Read the model definition and answer for the solid it produces. Units are mm, in the model's axes. A direction names the side the tool comes from. Coordinates: 2 decimals unless noted, no trailing zeros. Loops run counter-clockwise (first coordinate to the right, second up) from the corner with the lowest first, then second, coordinate; pieces in that order, holes last. Notation, with made-up numbers: (-38.5, 63) -> (-34.5, 63) arc R25 ccw to (-34.5, 81) -> close; hole circle Ø6 at (-4, 57). An arc over 180 degrees is marked (long way). Answer as a JSON object with one key per item and string values. Group by question number.
Q1. Straight lines are drawn through the part: line 1 along Z through (x, y) = (2.5, 3.5); line 2 along Z through (x, y) = (0, 0.5); line 3 along Z through (x, y) = (0, 4.85). For each, find the intervals that lie inside material, in ascending order. Write a range as [from, to].
Q2. The part is cut by section A-A on x = 0. Write down the section's boundary in (y, z).
Q3. The part is cut by section B-B on z = -6.5. Write down the section's boundary in (x, y).
Q4. Determine the mould class of faces 1 (the cylindrical face through (-0.404, 4.021, -9.574)), 2 (the flat face through (3, 5.5, 5)), 3 (the flat face through (4, 2, 1)) for opening direction X: released by +X, released by -X, zero draft, split by the parting line, or undercut.
Q5. Each of these flat-tipped pins is pushed along its axis until it touches: P1, Ø3, axis at x = -1.5, z = 8.5, coming from the -Y side; P2, Ø1, axis at x = 0.5, z = 0, coming from the -Y side; P3, Ø2.5, axis at x = 1.5, z = -6, coming from the -Y side; P4, Ø1.8, axis at x = 0, z = -6.5, coming from the -Y side (1 decimal). Where does it stop, or does it pass through?
Q6. For faces 4 (the flat face through (0, 0, -4)), 5 (the flat face through (0, -4, 7)), 6 (the flat face through (0, 4.5, 9.5)), determine the directions among +Z, -Z, +X, -X, +Y, -Y from which every point of the face is accessible in a straight line to the end or side of a thin tool.
Autodesk Inventor part; units mm, degrees
ref_plane "YZ Plane" through (0, 0, 0) normal (1, 0, 0) x (0, 1, 0)
ref_plane "XZ Plane" through (0, 0, 0) normal (0, 1, 0) x (-1, 0, 0)
ref_plane "XY Plane" through (0, 0, 0) normal (0, 0, 1) x (1, 0, 0)
sketch "Sketch1" plane through (0, 0, 0) normal (0, 1, 0) x (-1, 0, 0)
  line L0 (0, 10) -> (0, 10)
  line L1 (-4, 6) -> (-4, -6)
  line L2 (0, -10) -> (0, -10)
  line L3 (4, -6) -> (4, 6)
  line L4 (4, 10) -> (-4, -10) construction
  line L5 (-4, 10) -> (4, -10) construction
  circle A0 centre (0, -6.5) radius 1.5
  arc A1 (0, -10) -> (4, -6) centre (0, -6) ccw
  arc A2 (-4, -6) -> (0, -10) centre (0, -6) ccw
  arc A3 (4, 6) -> (0, 10) centre (0, 6) ccw
  arc A4 (0, 10) -> (-4, 6) centre (0, 6) ccw
  point P0 (0, 0)
  dimension "d0" = 8
  dimension "d1" = 20
  dimension "d2" = 3
  dimension "d3" = 3.5
  dimension "d4" = 4
extrude "Extrusion1" add sketch "Sketch1" along normal blind 5.5
sketch "Sketch2" plane through (0, 0, 0) normal (0, -1, 0) x (1, 0, 0)
  circle A0 centre (0, -6.5) radius 1.5 construction
  line L0 (-4, -6) -> (-4, 6) construction
  arc A1 (-4, -6) -> (4, -6) centre (0, -6) ccw construction
  line L1 (4, 6) -> (4, -6) construction
  arc A2 (4, 6) -> (-4, 6) centre (0, 6) ccw construction
  arc A3 (4, 6) -> (-4, 6) centre (0, 6) ccw
  arc A4 (4, 6) -> (-4, 6) centre (0, 5.2831) ccw
  point P0 (0, 0)
extrude "Extrusion2" cut sketch "Sketch2" against normal blind 4.5
sketch "Sketch4" plane through (0, 0, 0) normal (0, -1, 0) x (1, 0, 0)
  arc A0 (4, 6) -> (-4, 6) centre (0, 5.2831) ccw
  line L0 (-4, -6) -> (-4, 6)
  arc A1 (-4, -6) -> (4, -6) centre (0, -6) ccw
  line L1 (4, 6) -> (4, -6)
  circle A2 centre (0, -6.5) radius 1.5
  point P0 (0, 0)
extrude "Extrusion3" add sketch "Sketch4" along normal blind 4
sketch "Sketch6" plane through (0, -4, 0) normal (0, -1, 0) x (1, 0, 0)
  circle A0 centre (0, -6.5) radius 1.5
  arc A1 (-4, -6) -> (4, -6) centre (0, -6) ccw
  line L0 (4, 0) -> (4, -6)
  line L1 (4, 0) -> (-4, 0)
  arc A2 (-4, -6) -> (4, -6) centre (0, -6) ccw
  line L2 (-4, 0) -> (-4, -6)
  point P0 (0, 0)
extrude "Extrusion4" cut sketch "Sketch6" against normal blind 4
sketch "Sketch7" plane through (-4, 5.5, -6) normal (-1, 0, 0) x (0, 0, 1)
  line L0 (12, -9.5) -> (15.3469, -9.5)
  line L1 (6, -9.5) -> (12, -9.5)
  line L2 (12, -9.5) -> (6, -9.5)
  line L3 (6, -5.5) -> (6, -9.5)
  line L4 (6, -9.5) -> (6, -5.5)
  line L5 (12, -9.5) -> (12, -1)
  line L6 (6, -5.5) -> (12, -9.5)
extrude "Extrusion5" cut sketch "Sketch7" against normal through all
ref_plane "Work Plane1" through (-4, 0.1603, 8.7735) normal (0, -0.8321, -0.5547) x (1, 0, 0)
sketch "Sketch8" plane through (0, -4, 0) normal (0, -1, 0) x (1, 0, 0)
  line L0 (-4, 6) -> (4, 6) construction
  arc A0 (4, 6) -> (-4, 6) centre (0, 5.2831) ccw construction
  point P0 (0, 0)
  point P1 (0, 9.3469)
ref_plane "Work Plane3" through (-2, -4, 6) normal (0, 0.5547, -0.8321) x (1, 0, 0)
sketch "Sketch10" plane through (-2, -4, 6) normal (0, 0.5547, -0.8321) x (1, 0, 0)
  circle A0 centre (2, -4.3065) radius 3.55
  point P0 (2, 0)
  dimension "d18" = 7.1
extrude "Extrusion6" cut sketch "Sketch10" along normal blind 20 and the other way blind 10
sketch "Sketch11" plane through (0, 5.5, 0) normal (0, 1, 0) x (1, 0, 0)
  arc A0 (1.4864, 6.2983) -> (-1.4864, 6.2983) centre (0, 6.5) ccw construction
  circle A1 centre (0, 6.5) radius 3.1
  point P0 (0, 0)
  dimension "d23" = 6.2
extrude "Extrusion7" cut sketch "Sketch11" against normal blind 3
chamfer "Chamfer1" distance 1 angle 45 1 edges at (1.5, 2.5, -6.5)
properties part number "cable_cap"
Final values:
{
 "1": {"line 1": "z = [-9.12, -8.33], [-4.67, -2.03], [7.06, 8.49]", "line 2": "z = [-10, -8], [-5, 0.61]", "line 3": "z = [-10, -9.6], [6.89, 10]"},
 "2": {"outline": "(-4, 6) -> (0, 0) -> (0, -5) -> (1.5, -5) -> (2.5, -4) -> (2.5, -3.4) -> (3.18, -3.4) -> (-4, 7.36) -> close; (0, -10) -> (5.5, -10) -> (5.5, -9.6) -> (2.5, -9.6) -> (2.5, -9) -> (1.5, -8) -> (0, -8) -> close; (3.21, 9.35) -> (5.5, 5.91) -> (5.5, 10) -> (4.5, 10) -> (4.5, 9.35) -> close"},
 "3": {"outline": "(-3.97, 0) -> (-1.5, 0) -> (-1.5, 1.5) -> (-2.5, 2.5) -> (-3.1, 2.5) -> (-3.1, 5.5) -> (-3.97, 5.5) -> close; (1.5, 0) -> (3.97, 0) -> (3.97, 5.5) -> (3.1, 5.5) -> (3.1, 2.5) -> (2.5, 2.5) -> (1.5, 1.5) -> close"},
 "4": {"face 1": "undercut", "face 2": "zero draft", "face 3": "released by +X"},
 "5": {"P1": "stops at y = -4", "P2": "stops at y = -0.33", "P3": "stops at y = 0", "P4": "passes through"},
 "6": {"face 4": "-Z, +X, -X, -Y", "face 5": "+Z, -Z, +X, -X, -Y", "face 6": "+Z, -Y"}
}
